from build123d import *

# Parameters (mm, degrees)
BOSS_EXTRUDE1_DEPTH           = 6
M3_CLEARANCE_HOLE1_D          = 3.2
SKETCH7_R                     = 2.75
CUT_EXTRUDE1_DEPTH            = 3.8
CUT_EXTRUDE1_DRAFT            = 3
CUT_EXTRUDE1_PROFILE_2_DEPTH  = 3.8
CUT_EXTRUDE1_PROFILE_2_DRAFT  = 3
BOSS_EXTRUDE2_DEPTH           = 6
CBORE_FOR_M4_SHCS1_AT_2_COUNT = 2
CBORE_FOR_M4_SHCS1_AT_2_PITCH = 46.5


with BuildPart() as part:
    # Sketch1 → Boss-Extrude1 (new body)
    with BuildSketch(Plane(origin=(0, 0, 0), x_dir=(1, 0, 0), z_dir=(0, 1, 0))):
        with BuildLine():
            Line((-12.5, -4.75), (12.5, -4.75))
            ThreePointArc((12.5, -4.75), (17.25, 0), (12.5, 4.75))
            Line((12.5, 4.75), (12.5, 9.75))
            Line((12.5, 9.75), (-12.5, 9.75))
            Line((-12.5, 9.75), (-12.5, 4.75))
            ThreePointArc((-12.5, 4.75), (-17.25, 0), (-12.5, -4.75))
        make_face()
    extrude(amount=-BOSS_EXTRUDE1_DEPTH)

    # M3 Clearance Hole1 (through all)
    with Locations(Plane(origin=(0, -6, 0), x_dir=(-1, 0, 0), z_dir=(0, -1, 0))):
        with Locations((12.5, 0), (-12.5, 0)):
            Hole(M3_CLEARANCE_HOLE1_D / 2)


with BuildPart() as cut_extrude1_tool:
    # Sketch7 → Cut-Extrude1 (with draft: the straight prism first)
    with BuildSketch(Plane(origin=(0, -6, 0), x_dir=(-1, 0, 0), z_dir=(0, 1, 0))):
        with Locations((12.5, 0)):
            Circle(SKETCH7_R)
    extrude(amount=CUT_EXTRUDE1_DEPTH)
    # Cut-Extrude1: the draft: its side faces are tilted about the plane it starts from
    cut_extrude1_sides = [cut_extrude1_tool.faces().sort_by_distance(p)[0] for p in [
        (-9.75, -4.1, 0),
    ]]
    draft(cut_extrude1_sides, Plane(origin=(0, -6, 0), x_dir=(-1, 0, 0), z_dir=(0, 1, 0)), CUT_EXTRUDE1_DRAFT)


with BuildPart() as part_1:
    add(part.part)

    # Cut-Extrude1: cut by cut_extrude1_tool
    add(cut_extrude1_tool.part, mode=Mode.SUBTRACT)


with BuildPart() as cut_extrude1_profile_2_tool:
    # Sketch7 → Cut-Extrude1 profile 2 (with draft: the straight prism first)
    with BuildSketch(Plane(origin=(0, -6, 0), x_dir=(-1, 0, 0), z_dir=(0, 1, 0))):
        with Locations((-12.5, 0)):
            Circle(SKETCH7_R)
    extrude(amount=CUT_EXTRUDE1_PROFILE_2_DEPTH)
    # Cut-Extrude1 profile 2: the draft: its side faces are tilted about the plane it starts from
    cut_extrude1_profile_2_sides = [cut_extrude1_profile_2_tool.faces().sort_by_distance(p)[0] for p in [
        (15.25, -4.1, 0),
    ]]
    draft(cut_extrude1_profile_2_sides, Plane(origin=(0, -6, 0), x_dir=(-1, 0, 0), z_dir=(0, 1, 0)), CUT_EXTRUDE1_PROFILE_2_DRAFT)


with BuildPart() as part_2:
    add(part_1.part)

    # Cut-Extrude1 profile 2: cut by cut_extrude1_profile_2_tool
    add(cut_extrude1_profile_2_tool.part, mode=Mode.SUBTRACT)

    # Sketch4 → Boss-Extrude2 (add)
    with BuildSketch(Plane(origin=(0, 0, -9.75), x_dir=(-1, 0, 0), z_dir=(0, 0, -1))):
        with BuildLine():
            Line((23.25, 4.1), (-23.25, 4.1))
            ThreePointArc((-23.25, 4.1), (-27.99341649, 0.68113883), (-26.25, -4.9))
            ThreePointArc((-26.25, -4.9), (-24.689252713, -5.717758139), (-22.95, -6))
            Line((-22.95, -6), (22.95, -6))
            ThreePointArc((22.95, -6), (24.689252713, -5.717758139), (26.25, -4.9))
            ThreePointArc((26.25, -4.9), (27.99341649, 0.68113883), (23.25, 4.1))
        make_face()
    extrude(amount=BOSS_EXTRUDE2_DEPTH)

    # Sketch9 → CBORE for M4 SHCS1 (revolve, cut)
    with BuildSketch(Plane(origin=(23.25, -0.9, -9.75), x_dir=(0, -1, 0), z_dir=(1, 0, 0))):
        Polygon((0, 0), (0, 11.351936393), (2.25, 10), (2.25, 4), (4, 4), (4, 0.025), (4.025, 0), align=None)
    cbore_for_m4_shcs1 = revolve(axis=Axis((23.25, -0.9, -3.4), (0, 0, -1)), mode=Mode.SUBTRACT)

    # CBORE for M4 SHCS1 at 2: CBORE for M4 SHCS1 ×2
    with Locations(*[(-i * CBORE_FOR_M4_SHCS1_AT_2_PITCH, 0, 0) for i in range(1, CBORE_FOR_M4_SHCS1_AT_2_COUNT)]):
        add(cbore_for_m4_shcs1, mode=Mode.SUBTRACT)


solid = part_2.part
Geometry: final body of the model. Coordinates: model frame, mm. A direction names the side the tool comes from. Round coordinates to 2 decimals unless told otherwise and drop trailing zeros. Loops run counter-clockwise (first coordinate to the right, second up) from the corner with the lowest first, then second, coordinate; pieces in that order, holes last. Notation, with made-up numbers: M 19,21.25 L 35,21.25 A7 ccw 35,32.25 Z; hole C -13.5,1.25 d10. An arc over 180 degrees is marked long. Put each result on its own line as item: value. Start each with the question number.
(1) Section query A-A (y = -0.9). State how many separate pieces and enclosed holes the cut face has, then the cut area to 3 significant figures.
(2) Section query D-D (z = -8.5). Return loops of the section in (x, y), then the cut area to 3 significant figures.
(3) Draft query along Z for faces 4 (the face through (25, 1, -13.75)), 5 (the face through (11, -2.2, 1)), 6 (the face through (-24.666, -5.726, -12.708)). Return one class per face: +Z half, -Z half, draft (parallel to the pull), parting line (faces both ways), or undercut.
(4) Set-up query: faces 1 (the face through (0, 0, -3)), 2 (the face through (19.284, -0.379, -11.735)), 3 (the face through (-12.5, -3, -7)). Return all of +Z, -Z, +X, -X, +Y, -Y with unobstructed straight access to the full face (end or side cutting, diameter ignored); none if empty.
(5) Section query C-C (x = 16). Return loops of the section in (y, z).
(6) Section query B-B (z = -14.25). Return loops of the section in (x, y), then the cut area to 3 significant figures.
(7) Contact query for flat-ended pins moving along their axis: pin 1 Ø4 at (x, z) = (12.5, 0) entering from -Y; pin 2 Ø2.5 at (x, y) = (-23.25, -0.9) entering from +Z; pin 3 Ø4 at (y, z) = (0.5, -3.5) entering from -X; pin 4 Ø3 at (x, y) = (-20, -0.5) entering from +Z. Output: stop coordinate, or through.
(8) Material intervals for line 1 along X through (y, z) = (-0.9, -15.3); line 2 along Y through (x, z) = (-23.25, -12.6); line 3 along Y through (x, z) = (-23.25, -14.5), sorted ascending. Write a range as [from, to].
Findings below:
1. separate pieces: 3
1. enclosed holes: 2
1. area: 674 mm2
2. outline: M -12.5,-6 L 12.5,-6 L 12.5,0 L -12.5,0 Z
2. area: 150 mm2
3. face 4: +Z half
3. face 5: undercut
3. face 6: draft
4. face 1: +Z, +X, -X, +Y
4. face 2: +Z
4. face 3: -X, +Y, -Y
5. outline: M -6,-15.75 L 4.1,-15.75 L 4.1,-9.75 L -6,-9.75 Z; M -6,-3.21 L 0,-3.21 L 0,3.21 L -6,3.21 Z
6. outline: M -26.25,-4.9 A5.5 ccw -22.95,-6 L 22.95,-6 A5.5 ccw 26.25,-4.9 A5 ccw 23.25,4.1 L -23.25,4.1 A5 ccw Z; hole C -23.25,-0.9 d4.5; hole C 23.25,-0.9 d4.5
6. area: 517 mm2
7. pin 1: stops at y = -2.2
7. pin 2: passes through
7. pin 3: stops at x = -16.99
7. pin 4: stops at z = -9.75
8. line 1: x = [-28.25, -25.5], [-21, 21], [25.5, 28.25]
8. line 2: y = [-5.99, -4.9], [3.1, 4.1]
8. line 3: y = [-5.99, -3.15], [1.35, 4.1]
